from build123d import *

# Parameters (mm, degrees)
F0_W        = 23.3076866716
F0_H        = 113.6004934087
F1_DEPTH    = 25.4
F2_R        = 5.08
F3_T1_DEPTH = 45.72
F3_T3_DEPTH = 139.0004934087
F4_T1_DEPTH = 45.72
F4_T3_DEPTH = 139.0004934087
F5_T1_DEPTH = 38.5476866716


# Not quite as in the source:
# - a fillet or chamfer that OpenCascade refuses, or shapes differently, is made with other operations: its cross-section is extruded or revolved along the edge and cut away or added


with BuildPart() as f1:
    # F0 (on Front) → F1 (new body)
    with BuildSketch(Plane.XZ):
        with Locations((0, -1.4689718373)):
            Rectangle(F0_W, F0_H)
    extrude(amount=F1_DEPTH)

    # F2
    f2_edges = [f1.edges().sort_by_distance(p)[0] for p in [
        (0, -25.4, 55.331275),
        (-11.653843, -25.4, -1.468972),
        (0, -25.4, -58.269219),
        (11.653843, -25.4, -1.468972),
    ]]
    fillet(f2_edges, radius=F2_R)

    # F3: fillet of radius 5.08 on 4 edges, made by hand

    # F3_s2 → F3_t1 (cut)
    with BuildSketch(Plane.XZ.offset(-12.7)):
        with BuildLine():
            ThreePointArc((11.6538433358, -53.1892185417), (10.1659457842, -56.7813209901), (6.5738433358, -58.2692185417))
            Line((6.5738433358, -58.2692185417), (11.6538433358, -58.2692185417))
            Line((11.6538433358, -58.2692185417), (11.6538433358, -53.1892185417))
        make_face()
        with BuildLine():
            ThreePointArc((6.5738433358, 55.3312748671), (10.1659457842, 53.8433773155), (11.6538433358, 50.2512748671))
            Line((11.6538433358, 50.2512748671), (11.6538433358, 55.3312748671))
            Line((11.6538433358, 55.3312748671), (6.5738433358, 55.3312748671))
        make_face()
    extrude(amount=F3_T1_DEPTH, mode=Mode.SUBTRACT)

    # F3_s4 → F3_t3 (cut)
    with BuildSketch(Plane.XY.offset(-70.9692185417)):
        with BuildLine():
            ThreePointArc((11.6538433358, -5.08), (10.1659457842, -1.4878975516), (6.5738433358, 0))
            Line((6.5738433358, 0), (11.6538433358, 0))
            Line((11.6538433358, 0), (11.6538433358, -5.08))
        make_face()
    extrude(amount=F3_T3_DEPTH, mode=Mode.SUBTRACT)

    # F4: fillet of radius 5.08 on 4 edges, made by hand

    # F4_s2 → F4_t1 (cut)
    with BuildSketch(Plane.XZ.offset(-12.7)):
        with BuildLine():
            ThreePointArc((-6.5738433358, 55.3312748671), (-10.1659457842, 53.8433773155), (-11.6538433358, 50.2512748671))
            Line((-11.6538433358, 50.2512748671), (-11.6538433358, 55.3312748671))
            Line((-11.6538433358, 55.3312748671), (-6.5738433358, 55.3312748671))
        make_face()
        with BuildLine():
            ThreePointArc((-11.6538433358, -53.1892185417), (-10.1659457842, -56.7813209901), (-6.5738433358, -58.2692185417))
            Line((-6.5738433358, -58.2692185417), (-11.6538433358, -58.2692185417))
            Line((-11.6538433358, -58.2692185417), (-11.6538433358, -53.1892185417))
        make_face()
    extrude(amount=F4_T1_DEPTH, mode=Mode.SUBTRACT)

    # F4_s4 → F4_t3 (cut)
    with BuildSketch(Plane.XY.offset(-70.9692185417)):
        with BuildLine():
            ThreePointArc((-6.5738433358, 0), (-10.1659457842, -1.4878975516), (-11.6538433358, -5.08))
            Line((-11.6538433358, -5.08), (-11.6538433358, 0))
            Line((-11.6538433358, 0), (-6.5738433358, 0))
        make_face()
    extrude(amount=F4_T3_DEPTH, mode=Mode.SUBTRACT)

    # F5: fillet of radius 5.08 on 4 edges, made by hand

    # F5_s2 → F5_t1 (cut)
    with BuildSketch(Plane.YZ.offset(-19.2738433358)):
        with BuildLine():
            ThreePointArc((-5.08, 55.3312748671), (-1.4878975516, 53.8433773155), (0, 50.2512748671))
            Line((0, 50.2512748671), (0, 55.3312748671))
            Line((0, 55.3312748671), (-5.08, 55.3312748671))
        make_face()
        with BuildLine():
            ThreePointArc((0, -53.1892185417), (-1.4878975516, -56.7813209901), (-5.08, -58.2692185417))
            Line((-5.08, -58.2692185417), (0, -58.2692185417))
            Line((0, -58.2692185417), (0, -53.1892185417))
        make_face()
    extrude(amount=F5_T1_DEPTH, mode=Mode.SUBTRACT)


solid = f1.part
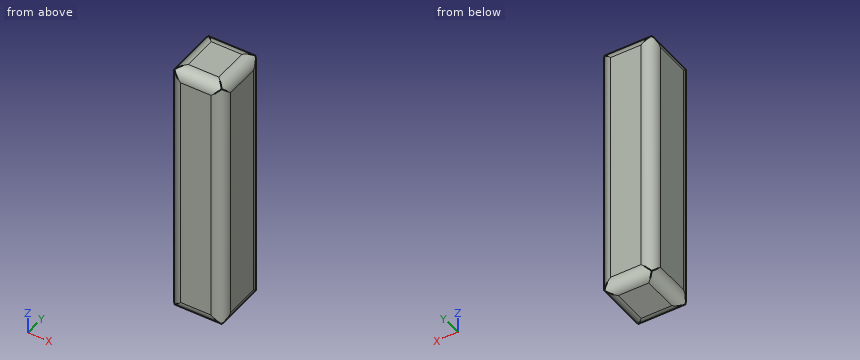
Can you work these out from the model? Positions are in its coordinate system, mm. Coordinates: 2 decimals unless noted, no trailing zeros. Write each loop counter-clockwise with the first axis right and the second up, starting at its lowest first coordinate (ties: lowest second). Pieces come first, ordered by that corner, then holes. Notation, with made-up numbers: (-38, 34.5) -> (-2, 34.5) arc R24 ccw to (-2, 65.5) -> close; hole circle Ø4 at (-7, 58.25). An arc over 180 degrees is marked (long way). Write each question's results on one line, items separated by ' | '. Start each with the question number.
Item 1: If we section it at A-A, the plane z = 23: Write out the boundary of the cut face in (x, y).
Item 2: I'm going to push flat-ended pins straight in: P1, Ø1.5, axis at x = 5, y = -22, coming from the -Z side; P2, Ø5, axis at x = -9.5, y = -14.5, coming from the -Z side. Where does each tip first touch, or does it pass through?
Item 3: If we section it at B-B, the plane x = -8.25: Write out the boundary of the cut face in (y, z), and give its area (3 significant figures).
Item 4: Please list where these lines run through material, in increasing order: probe 1 along Z at (x, y) = (-7, -20); probe 2 along Z at (x, y) = (-8.5, -1.5); probe 3 along Y at (x, z) = (10.5, 2).
Answer block:
1) outline: (-11.65, -20.32) arc R5.08 ccw to (-6.57, -25.4) -> (6.57, -25.4) arc R5.08 ccw to (11.65, -20.32) -> (11.65, -5.08) arc R5.08 ccw to (6.57, 0) -> (-6.57, 0) arc R5.08 ccw to (-11.65, -5.08) -> close
2) P1: z = -58.18 | P2: z = -58.25
3) outline: (-25.12, -54.87) arc R5.08 ccw to (-22, -57.98) -> (-3.4, -57.98) arc R5.08 ccw to (-0.28, -54.87) -> (-0.28, 51.93) arc R5.08 ccw to (-3.4, 55.05) -> (-22, 55.05) arc R5.08 ccw to (-25.12, 51.93) -> close | area: 2,790 mm²
4) probe 1: -58.25 to 55.31 | probe 2: -56.79 to 53.86 | probe 3: -23.54 to -1.86
